Work out the finished part from the listing and answer in its coordinate system (mm). A direction names the side the tool comes from. Round coordinates to 2 decimals unless told otherwise and drop trailing zeros. One line per item, written item: value. Start each with the question number.
Q1. A tool of negligible diameter and unlimited length cuts with its end or side. For faces 1 (the flat face through (-88.846, -13, -13)), 2 (the flat face through (128.846, 0, 0)), 3 (the flat face through (88.846, -13, -13)), from which of +Z, -Z, +X, -X, +Y, -Y can it reach the whole face along a straight path? Write none if from no direction.
Q2. Given pin 1 Ø6 at (y, z) = (-7, 22) entering from +X; pin 2 Ø3 at (x, y) = (-37, 9) entering from -Z; pin 3 Ø8 at (x, y) = (17, -5.5) entering from -Z, each flat-ended and moving along its own axis, determine where each tip first touches the part or whether it passes through.
Q3. Consider probe 1 along X at (y, z) = (1, 19.5); probe 2 along X at (y, z) = (-25.5, 1); probe 3 along Z at (x, y) = (-75.5, -1). Determine where each line is inside the solid, lowest interval first.
from build123d import *


with BuildPart() as f1:
    # F0 (on Front) → F1 (revolve)
    with BuildSketch(Plane.XZ):
        with BuildLine():
            Line((0, 9.6923084871), (0, 0))
            Line((0, 0), (128.8461439112, 0))
            Line((128.8461439112, 0), (128.8461439112, 17.5))
            Line((128.8461439112, 17.5), (88.8461439112, 17.5))
            Line((88.8461439112, 17.5), (88.8461439112, 30))
            Line((88.8461439112, 30), (68.1153744155, 30))
            add(Edge.make_bspline(
                [(0, 9.6923084871), (4.2903837959, 9.2833106214), (13.4700518004, 8.4082223307), (31.2065009966, 15.3510841597), (35.2364916061, 30.6873308582), (53.225939561, 30.2545752312), (63.1567054052, 30.0847818821), (68.1153744155, 30)],
                knots=[0, 0, 0, 0, 0.1895589819, 0.4055787556, 0.5938281877, 0.7971886952, 1, 1, 1, 1], degree=3))
        make_face()
    revolve(axis=Axis((64.4230719556, 0, 0), (-1, 0, 0)))

    # F2: F1 across face


with BuildPart() as f1_1:
    add(f1.part)
    add(f1.part.mirror(Plane(origin=(0, 0, 0), x_dir=(0, -1, 0), z_dir=(-1, 0, 0))))


solid = f1_1.part
The answers:
1. face 1: -X
1. face 2: +Z, -Z, +X, +Y, -Y
1. face 3: +X
2. pin 1: x = 88.85
2. pin 2: z = -27.36
2. pin 3: z = -11.06
3. probe 1: -88.85 to -31.14, 31.14 to 88.85
3. probe 2: -88.85 to -34.88, 34.88 to 88.85
3. probe 3: -29.98 to 29.98
